Here's the drawing with two shaded views (mm, measured from the low corner). I have some questions. A direction names the side the tool comes from. Round coordinates to 2 decimals unless told otherwise and drop trailing zeros. Loops run counter-clockwise (first coordinate to the right, second up) from the corner with the lowest first, then second, coordinate; pieces in that order, holes last.
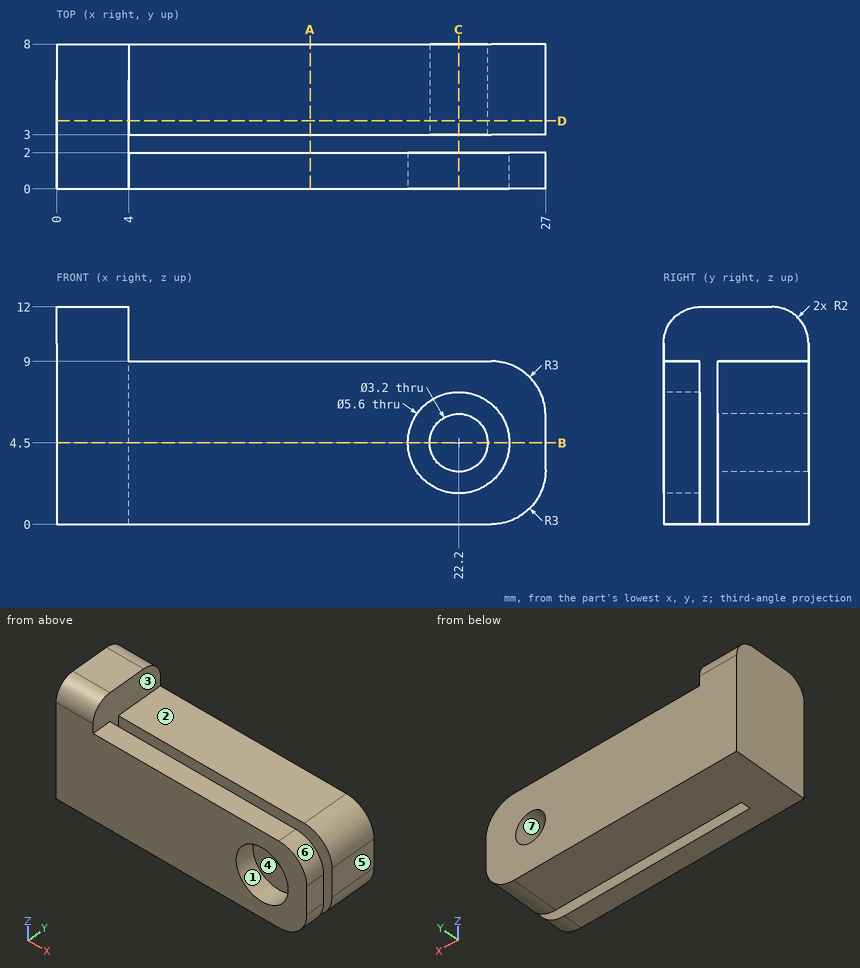
Item 1: We'd pull the mould along Z, two halves only. Please class the marked faces 5, 6 and 7: released by +Z, released by -Z, zero draft, split by the parting line, or undercut.
Results list:
face 5: zero draft
face 6: released by +Z
face 7: undercut
Item 2: If we section it at C-C, the plane x = 22.2: Please give me the cut outline in (y, z), then the cut area to 3 significant figures.
Results list:
outline: (0, 0) - (2, 0) - (2, 1.7) - (0, 1.7) - close; (0, 7.3) - (2, 7.3) - (2, 9) - (0, 9) - close; (3, 0) - (8, 0) - (8, 2.9) - (3, 2.9) - close; (3, 6.1) - (8, 6.1) - (8, 9) - (3, 9) - close
area: 35.8 mm2
Item 3: Will these pins go through, and if not, where does the flat tip stop? pin 1 (1.6 mm diameter, centred on x = 13, y = 1, fed in from +Z); pin 2 (3.5 mm diameter, centred on x = 22.2, z = 4.5, fed in from -Y).
Results list:
pin 1: stops at z = 9
pin 2: stops at y = 3
Item 4: If we section it at D-D, the plane y = 3.75: Please give me the cut outline in (x, z).
Results list:
outline: (0, 0) - (24, 0) arc R3 ccw to (27, 3) - (27, 6) arc R3 ccw to (24, 9) - (4, 9) - (4, 12) - (0, 12) - close; hole circle Ø3.2 at (22.2, 4.5)
Item 5: If we section it at A-A, the plane x = 14: Please give me the cut outline in (y, z).
Results list:
outline: (0, 0) - (2, 0) - (2, 9) - (0, 9) - close; (3, 0) - (8, 0) - (8, 9) - (3, 9) - close
Item 6: If we section it at B-B, the plane z = 4.5: Please give me the cut outline in (x, y), then the cut area to 3 significant figures.
Results list:
outline: (0, 0) - (19.4, 0) - (19.4, 2) - (4, 2) - (4, 3) - (20.6, 3) - (20.6, 8) - (0, 8) - close; (23.8, 3) - (27, 3) - (27, 8) - (23.8, 8) - close; (25, 0) - (27, 0) - (27, 2) - (25, 2) - close
area: 166 mm2
Item 7: For the marked faces 1, 2, 3 and 4, which set-ups out of +Z, -Z, +X, -X, +Y, -Y let a thin tool reach every point of the face, with its end or its side?
Results list:
face 1: -Y
face 2: +Z, +X, +Y, -Y
face 3: +Z, +X
face 4: +Z, -Z, +X
Item 8: If I drill on line 1 along Y through (x, z) = (16.5, 4.75); line 2 along X through (y, z) = (1.2, 4.5); line 3 along Z through (x, y) = (22.2, 5.95), over which ranges is the centre line in solid material (lowest first)?
Results list:
line 1: y = 0 to 2, 3 to 8
line 2: x = 0 to 19.4, 25 to 27
line 3: z = 0 to 2.9, 6.1 to 9
